Print and shaded views of the part. All mm, measured from the part's lowest x, y and z. A direction names the side the tool comes from. Coordinates: 2 decimals unless noted, no trailing zeros. Order: outer loops, then holes, each group sorted by start corner. A loop starts at its lowest first (then second) coordinate and runs counter-clockwise, first axis right, second up. Notation, with made-up numbers: (72.25, -25) -> (87.25, -25) arc R9 cw to (87.25, -10) -> close; hole circle Ø1 at (-12, 14). An arc over 180 degrees is marked (long way). Return JSON: item names as keys, results as strings. Group by question number.
1) Cut at D-D (y = 12). Write the cut outline in (x, z).
2) Probe line 1 (X direction, y = 8.5, z = 9); line 2 (Z direction, x = 4, y = 7.25); line 3 (Y direction, x = 2, z = 1.75). List the from-to ranges inside material, lowest first.
3) Which spindle directions (+Z, -Z, +X, -X, +Y, -Y) get a long thin tool onto all of the face, cutting with end or side? Do the marked faces 5 and 6. Say none if no direction does.
4) Cut at C-C (x = 25.5). Write the cut outline in (y, z).
5) Cut at A-A (y = 3.5). Write the cut outline in (x, z).
6) Flat gauge pins, fed straight in: pin 1 (1.5 mm diameter, centred on x = 12, z = 6.5, fed in from +Y); pin 2 (12 mm diameter, centred on x = 22.5, z = 5.5, fed in from +Y). Where does each tip first touch, or does it go through?
7) Pull direction X, two halves, no side cores. Call the marked faces 1, 2, 3 and 4: +X half, -X half, draft (parallel to the pull), parting line (faces both ways), or undercut.
8) Cut at B-B (z = 19.5). Write the cut outline in (x, y), and give its area (3 significant figures).
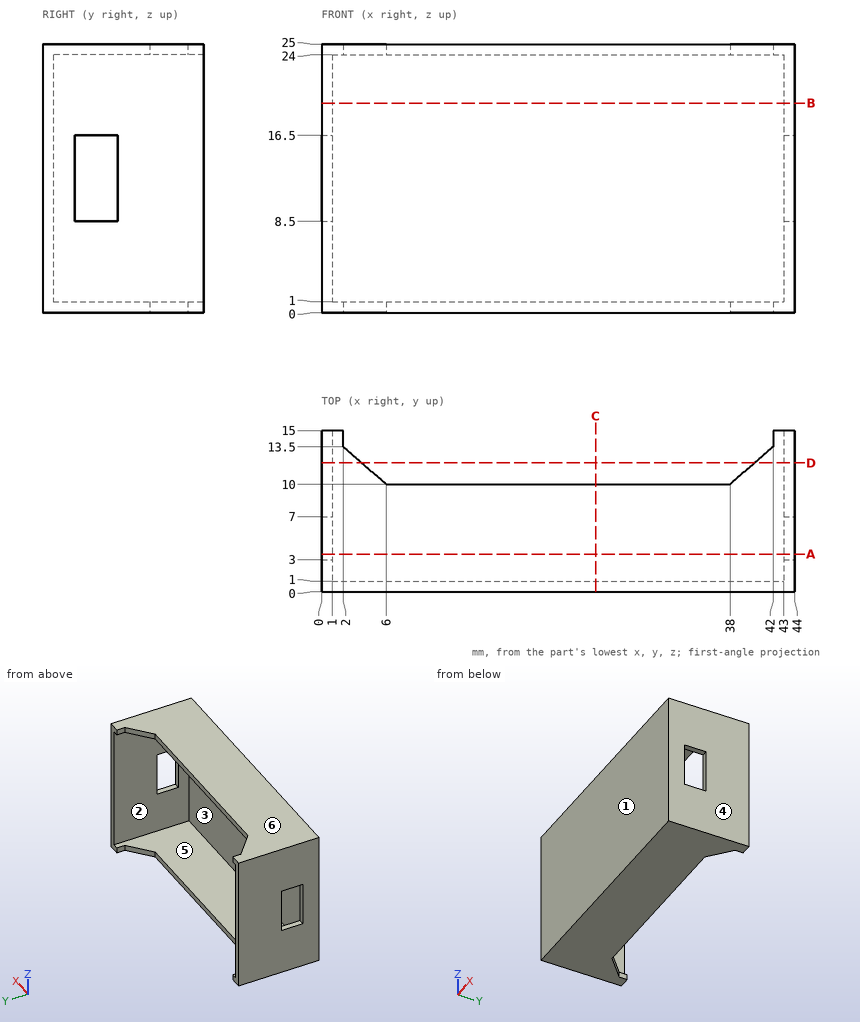
Answers below:
{
 "1": {"outline": "(0, 0) -> (3.71, 0) -> (3.71, 1) -> (1, 1) -> (1, 24) -> (3.71, 24) -> (3.71, 25) -> (0, 25) -> close; (40.29, 0) -> (44, 0) -> (44, 25) -> (40.29, 25) -> (40.29, 24) -> (43, 24) -> (43, 1) -> (40.29, 1) -> close"},
 "2": {"line 1": "x = 0 to 1, 43 to 44", "line 2": "z = 0 to 1, 24 to 25", "line 3": "y = 0 to 1"},
 "3": {"face 5": "+Y", "face 6": "+Z, +X, -X, +Y, -Y"},
 "4": {"outline": "(0, 0) -> (10, 0) -> (10, 1) -> (1, 1) -> (1, 24) -> (10, 24) -> (10, 25) -> (0, 25) -> close"},
 "5": {"outline": "(0, 0) -> (44, 0) -> (44, 8.5) -> (43, 8.5) -> (43, 1) -> (1, 1) -> (1, 8.5) -> (0, 8.5) -> close; (0, 16.5) -> (1, 16.5) -> (1, 24) -> (43, 24) -> (43, 16.5) -> (44, 16.5) -> (44, 25) -> (0, 25) -> close"},
 "6": {"pin 1": "stops at y = 1", "pin 2": "stops at y = 10"},
 "7": {"face 1": "draft", "face 2": "undercut", "face 3": "undercut", "face 4": "+X half"},
 "8": {"outline": "(0, 0) -> (44, 0) -> (44, 15) -> (43, 15) -> (43, 1) -> (1, 1) -> (1, 15) -> (0, 15) -> close", "area": "72.0 mm^2"}
}
